For this review, take the finished solid that the model builds, in its own axes (mm). A direction names the side the tool comes from. Round coordinates to 2 decimals unless told otherwise and drop trailing zeros. Write each loop counter-clockwise with the first axis right and the second up, starting at its lowest first coordinate (ties: lowest second). Pieces come first, ordered by that corner, then holes. Notation, with made-up numbers: (-36, 79) -> (1, 79) arc R9 ccw to (1, 83) -> close; hole circle Ø9 at (79, 48.5). An arc over 180 degrees is marked (long way). Answer as CSV lines item,"result". Start each with the question number.
Item 1: Wall thickness on probe 1 along Z at (x, y) = (25.5, 4.75); probe 2 along X at (y, z) = (6.25, 6); probe 3 along X at (y, z) = (5, 7): over which ranges is each line inside the solid? List them lowest first. Write a range as from..to.
Item 2: Mouldability with a two-part tool opening along X and no side actions: class faces 1 (the cylindrical face through (-15.02, 3.2, -47.69)), 2 (the cylindrical face through (23.174, 2.613, 25.642)), 3 (the flat face through (-12, 0, 23)), 4 (the flat face through (12.675, 3.295, -21.55)) as +X half, -X half, draft (parallel to the pull), parting line (faces both ways), or undercut.
Item 3: Take a section at B-B on y = 1.5. Give the boundary of the cut face in (x, z), then the cut area to 3 significant figures.
Item 4: Take a section at A-A on z = 0. Give the boundary of the cut face in (x, y).
Item 5: Machinability: for faces 5 (the flat face through (25, 3, 0)), 6 (the flat face through (0, 2.5, 35)), 7 (the flat face through (-12, 6.5, 23)), which of the approach directions +Z, -Z, +X, -X, +Y, -Y give a long, thin tool a straight path to every point of the face, cutting with its end or side? Answer none if there is none.
Item 6: Take a section at C-C on x = 17. Give the boundary of the cut face in (y, z).
Item 7: Take a section at D-D on z = 25.5. Count the separate pieces of the cut face and the enclosed holes in it, then the cut area to 3 significant figures.
Item 8: For pin 1 Ø1 at (x, y) = (-28, 5) entering from +Z; pin 2 Ø1.5 at (x, y) = (37.5, 1.5) entering from +Z; pin 3 Ø1.5 at (x, z) = (23.5, 26.5) entering from +Y; pin 4 Ø4 at (x, z) = (10, -25) entering from -Y, all flat-tipped, find the tip position at first contact; note any pin that passes through.
```python
from build123d import *

# Parameters (mm, degrees)
SKETCH1_R           = 50
SKETCH1_R_2         = 2.2
BOSS_EXTRUDE1_DEPTH = 6.5
BOSS_EXTRUDE2_START = -2
SKETCH1_3_R         = 2.2
BOSS_EXTRUDE2_DEPTH = 2
SKETCH2_R           = 5.5
CUT_EXTRUDE1_DEPTH  = 2.5
CUT_EXTRUDE2_DEPTH  = 10
CHAMFER1_SIZE       = 1.2


with BuildPart() as part:
    # Sketch1 → Boss-Extrude1 (new body)
    with BuildSketch(Plane(origin=(0, 0, 0), x_dir=(1, 0, 0), z_dir=(0, 1, 0))):
        with Locations(Location((0, 0, 0), (0, 0, 90))):
            Circle(SKETCH1_R)
        with Locations(Location((-25.355339059, 25.355339059, 0), (0, 0, 90))):
            Circle(SKETCH1_R_2, mode=Mode.SUBTRACT)
        with Locations(Location((25.355339059, 25.355339059, 0), (0, 0, 90))):
            Circle(SKETCH1_R_2, mode=Mode.SUBTRACT)
        with Locations(Location((-25.355339059, -25.355339059, 0), (0, 0, 90))):
            Circle(SKETCH1_R_2, mode=Mode.SUBTRACT)
        with Locations(Location((25.355339059, -25.355339059, 0), (0, 0, 90))):
            Circle(SKETCH1_R_2, mode=Mode.SUBTRACT)
    extrude(amount=BOSS_EXTRUDE1_DEPTH)

    # Sketch1_3 → Boss-Extrude2 (add)
    with BuildSketch(Plane(origin=(0, 0, 0), x_dir=(1, 0, 0), z_dir=(0, 1, 0)).offset(BOSS_EXTRUDE2_START)):
        with Locations(Location((25.355339059, -25.355339059, 0), (0, 0, 90))):
            Circle(SKETCH1_3_R)
        with Locations(Location((25.355339059, 25.355339059, 0), (0, 0, 90))):
            Circle(SKETCH1_3_R)
        with Locations(Location((-25.355339059, 25.355339059, 0), (0, 0, 90))):
            Circle(SKETCH1_3_R)
        with Locations(Location((-25.355339059, -25.355339059, 0), (0, 0, 90))):
            Circle(SKETCH1_3_R)
    extrude(amount=BOSS_EXTRUDE2_DEPTH)


with BuildPart() as boss_extrude2_kept_piece:
    # of the separate pieces the step leaves, the one the design keeps (boss_extrude2_pieces_kept)
    add(part.part.solids().sort_by_distance((0, 0, -50))[0])

    # Sketch2 → Cut-Extrude1 (cut)
    with BuildSketch(Plane.XZ):
        with Locations(Location((0, 35.355339059, 0), (0, 0, 270))):
            Circle(SKETCH2_R)
    extrude(amount=-CUT_EXTRUDE1_DEPTH, mode=Mode.SUBTRACT)

    # Sketch3 → Cut-Extrude2 (cut)
    with BuildSketch(Plane(origin=(0, 6.5, 0), x_dir=(1, 0, 0), z_dir=(0, 1, 0))):
        Polygon((0, 28.867513459), (-25, 14.43375673), (-25, -14.43375673), (0, -28.867513459), (25, -14.43375673), (25, 14.43375673), align=None)
    extrude(amount=-CUT_EXTRUDE2_DEPTH, mode=Mode.SUBTRACT)

    # Chamfer1
    chamfer1_edges = [boss_extrude2_kept_piece.edges().sort_by_distance(p)[0] for p in [
        (25.355339059, 6.5, 27.555339059),
        (25.355339059, 6.5, -23.155339059),
        (-25.355339059, 6.5, -23.155339059),
        (-25.355339059, 6.5, 27.555339059),
    ]]
    chamfer(chamfer1_edges, length=CHAMFER1_SIZE)


solid = boss_extrude2_kept_piece.part
```
Output values:
1,probe 1,"z = -43.01..-27.55, -23.16..23.16, 27.55..43.01"
1,probe 2,"x = -49.64..-25, 25..49.64"
1,probe 3,"x = -49.51..-25, 25..49.51"
2,face 1,"parting line"
2,face 2,"undercut"
2,face 3,"draft"
2,face 4,"undercut"
3,outline,"circle Ø100 at (0, 0); hole circle Ø4.4 at (-25.36, -25.36); hole circle Ø4.4 at (-25.36, 25.36); hole (-25, -14.43) -> (0, -28.87) -> (25, -14.43) -> (25, 14.43) -> (0, 28.87) -> (-25, 14.43) -> close; hole circle Ø11 at (0, 35.36); hole circle Ø4.4 at (25.36, -25.36); hole circle Ø4.4 at (25.36, 25.36)"
3,area,"5,530 mm^2"
4,outline,"(-50, 0) -> (-25, 0) -> (-25, 6.5) -> (-50, 6.5) -> close; (25, 0) -> (50, 0) -> (50, 6.5) -> (25, 6.5) -> close"
5,face 5,"+Y, -Y"
5,face 6,"-Y"
5,face 7,"+Z, -Z, +X, -X, +Y"
6,outline,"(0, -47.02) -> (6.5, -47.02) -> (6.5, -19.05) -> (0, -19.05) -> close; (0, 19.05) -> (6.5, 19.05) -> (6.5, 47.02) -> (0, 47.02) -> close"
7,separate pieces,"4"
7,enclosed holes,"0"
7,area,"423 mm^2"
8,pin 1,"stops at z = 41.76"
8,pin 2,"stops at z = 33.9"
8,pin 3,"stops at y = 6.03"
8,pin 4,"stops at y = 0"
